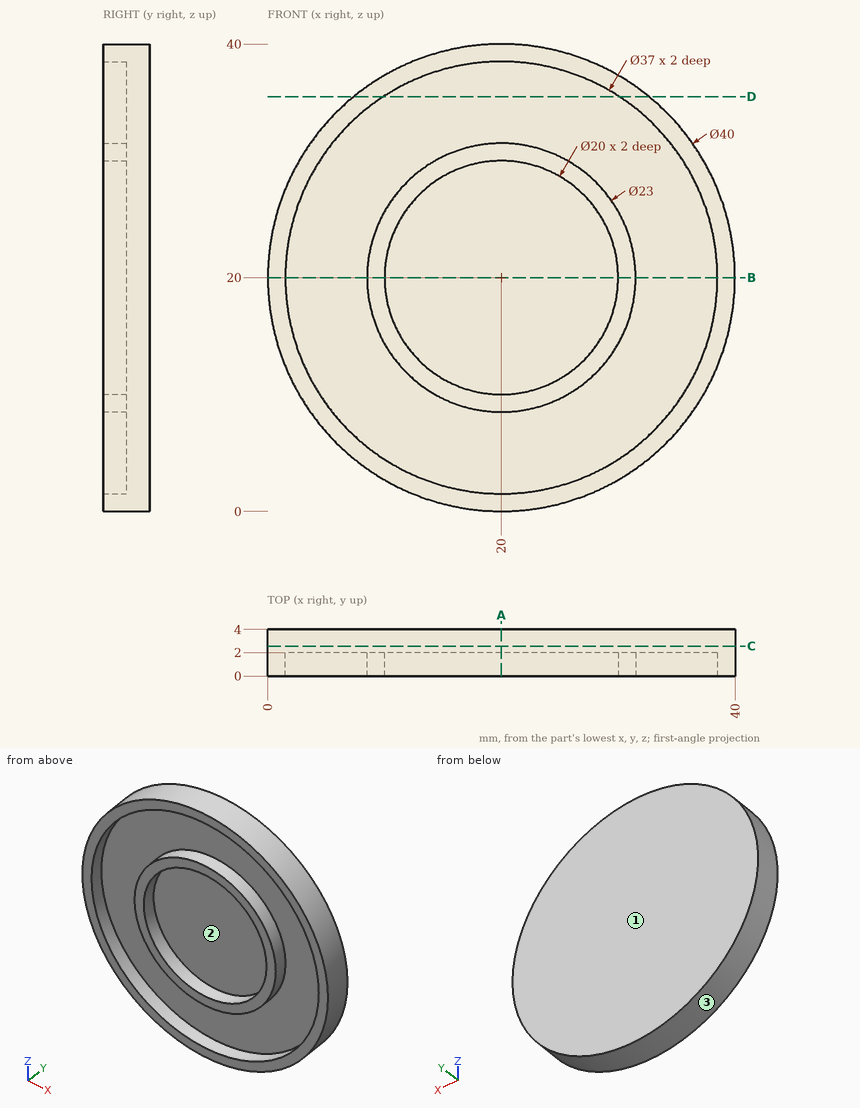
Here's the drawing with two shaded views (mm, measured from the low corner). I have some questions. Coordinates: 2 decimals unless noted, no trailing zeros. Write each loop counter-clockwise with the first axis right and the second up, starting at its lowest first coordinate (ties: lowest second). Pieces come first, ordered by that corner, then holes. Notation, with made-up numbers: (84, 18.5) - (137, 18.5) arc R12 ccw to (137, 37.5) - close; hole circle Ø9 at (17.25, 33). An arc over 180 degrees is marked (long way). Return JSON: item names as keys, results as strings.
Q1. If we section it at C-C (y = 2.55): Please give me the cut outline in (x, z).
Computed values:
{"outline": "circle Ø40 at (20, 20)"}
Q2. If we section it at A-A (x = 20): Please give me the cut outline in (y, z).
Computed values:
{"outline": "(0, 0) - (4, 0) - (4, 40) - (0, 40) - (0, 38.5) - (2, 38.5) - (2, 31.5) - (0, 31.5) - (0, 30) - (2, 30) - (2, 10) - (0, 10) - (0, 8.5) - (2, 8.5) - (2, 1.5) - (0, 1.5) - close"}
Q3. If we section it at B-B (z = 20): Please give me the cut outline in (x, y), then the cut area to 3 significant figures.
Computed values:
{"outline": "(0, 0) - (1.5, 0) - (1.5, 2) - (8.5, 2) - (8.5, 0) - (10, 0) - (10, 2) - (30, 2) - (30, 0) - (31.5, 0) - (31.5, 2) - (38.5, 2) - (38.5, 0) - (40, 0) - (40, 4) - (0, 4) - close", "area": "92.0 mm2"}
Q4. Please list where these lines run through material, in increasing order: L1, parallel to Z at x = 20, y = 0.75; L2, parallel to Z at x = 27.5, y = 0.75; L3, parallel to Z at x = 9.5, y = 1.15. Write a range as from..to.
Computed values:
{"L1": "z = 0..1.5, 8.5..10, 30..31.5, 38.5..40", "L2": "z = 1.46..3.09, 11.28..13.39, 26.61..28.72, 36.91..38.54", "L3": "z = 2.98..4.77, 15.31..24.69, 35.23..37.02"}
Q5. Thinking about a two-plate mould opening in X: for the marked faces 1, 2 and 3, which applies, +X half, -X half, draft (parallel to the pull), parting line (faces both ways), or undercut?
Computed values:
{"face 1": "draft", "face 2": "undercut", "face 3": "parting line"}
Q6. If we section it at D-D (z = 35.5): Please give me the cut outline in (x, y).
Computed values:
{"outline": "(7.36, 0) - (9.9, 0) - (9.9, 2) - (30.1, 2) - (30.1, 0) - (32.64, 0) - (32.64, 4) - (7.36, 4) - close"}
Q7. I'm going to push flat-ended pins straight in: pin 1 Ø1 at (x, y) = (6.5, 2.5) entering from +Z; pin 2 Ø1 at (x, y) = (16, 0.5) entering from +Z; pin 3 Ø1 at (y, z) = (0.5, 22.5) entering from +X; pin 4 Ø16 at (x, z) = (18, 16) entering from -Y. Where does each tip first touch, or does it pass through?
Computed values:
{"pin 1": "stops at z = 35.2", "pin 2": "stops at z = 39.69", "pin 3": "stops at x = 39.9", "pin 4": "stops at y = 0"}
